Can you work these out from the model? Positions are in its coordinate system, mm. Face numbers are marked on the shaded views. A direction names the side the tool comes from. Coordinates: 2 decimals unless noted, no trailing zeros. Order: outer loops, then holes, each group sorted by start corner. A loop starts at its lowest first (then second) coordinate and runs counter-clockwise, first axis right, second up. Notation, with made-up numbers: (-2.5, 89) -> (20.5, 89) arc R34 ccw to (20.5, 125) -> close; hole circle Ø6 at (-34, 49). An arc over 180 degrees is marked (long way). Answer as CSV lines item,"result".
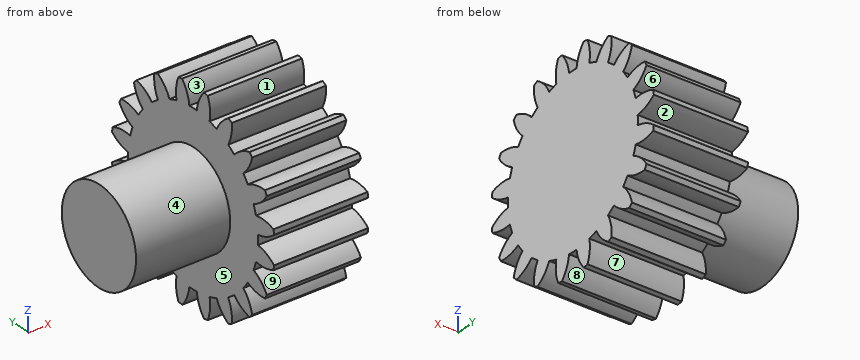
from build123d import *

# Parameters (mm, degrees)
BASPROSKE_W     = 10
BASPROSKE_H     = 11
TOOTHCUT_DEPTH  = 19.493242009
TEETHCUTS_COUNT = 20
TEETHCUTS_ANGLE = 342
BORSKE_R        = 0.5
BORE_DEPTH      = 50.0000508
SKETCH_1_R      = 5
EXTRUDE_1_DEPTH = 20


with BuildPart() as part:
    # BasProSke → Base-Revolve (revolve)
    with BuildSketch(Plane(origin=(0, 0, 0), x_dir=(1, 0, 0), z_dir=(0, 1, 0)), mode=Mode.PRIVATE) as base_revolve_sk:
        with Locations((5, 5.5)):
            Rectangle(BASPROSKE_W, BASPROSKE_H)
    revolve(base_revolve_sk.sketch.rotate(Axis((-10, 0, 0), (1, 0, 0)), 180), axis=Axis((-10, 0, 0), (1, 0, 0)))

    # TooCutSke → ToothCut (cut, through all)
    with BuildSketch(Plane(origin=(0, 0, 0), x_dir=(0, 0, -1), z_dir=(1, 0, 0))):
        with BuildLine():
            ThreePointArc((0.499924007, 8.734705318), (0, 8.749), (-0.499924007, 8.734705318))
            ThreePointArc((-0.499924007, 8.734705318), (-0.824302243, 9.905497836), (-1.485192705, 10.924909509))
            ThreePointArc((-1.485192705, 10.924909509), (0, 11.0254), (1.485192705, 10.924909509))
            ThreePointArc((1.485192705, 10.924909509), (0.824302243, 9.905497836), (0.499924007, 8.734705318))
        make_face()
    toothcut = extrude(amount=TOOTHCUT_DEPTH, mode=Mode.SUBTRACT)

    # TeethCuts: ToothCut ×20 about axis
    teethcuts_axis = Axis((-10, 0, 0), (1, 0, 0))
    for i in range(1, TEETHCUTS_COUNT):
        add(toothcut.rotate(teethcuts_axis, i * TEETHCUTS_ANGLE / (TEETHCUTS_COUNT - 1)), mode=Mode.SUBTRACT)

    # BorSke → Bore (cut, symmetric)
    with BuildSketch(Plane(origin=(0, 0, 0), x_dir=(0, 0, -1), z_dir=(1, 0, 0))):
        with Locations(Location((0, 0, 0), (0, 0, 180))):
            Circle(BORSKE_R)
    extrude(amount=BORE_DEPTH, both=True, mode=Mode.SUBTRACT)

    # 草图1 → 凸台-拉伸1 (add)
    with BuildSketch(Plane(origin=(10, 0, 0), x_dir=(0, 0, -1), z_dir=(1, 0, 0))):
        Circle(SKETCH_1_R)
    extrude(amount=-EXTRUDE_1_DEPTH)


solid = part.part
Q1. Which directions (+Z, -Z, +X, -X, +Y, -Y) give clear straight access to the entire face, cutting with the end or side of a thin tool? Please do the marked faces 5, 6, 7, 8 and 9.
Solution:
face 5,"-X"
face 6,"+X, -X, +Y"
face 7,"+X, -X"
face 8,"-Z, +X, -X"
face 9,"+X, -X, -Y"
Q2. Imagine slicing it at C-C (x = -3). List the corners of the cut face in (y, z) for me, and give its area (3 significant figures).
Solution:
outline,"circle Ø10 at (0, 0)"
area,"78.5 mm2"
Q3. For P1, Ø8, axis at x = 3.5, z = 5.5, coming from the -Y side; P2, Ø1.5, axis at y = -8.5, z = 3, coming from the -X side; P3, Ø2, axis at x = 0, z = -3.5, coming from the +Y side, each with a flat end and sliding along its axis, tell me the tip position at first contact or that it passes through.
Solution:
P1,"y = -10.9"
P2,"x = 0"
P3,"y = 9.75"
Q4. If I drill on line 1 (Z direction, x = 3.5, y = 9.5); line 2 (X direction, y = 3.5, z = 4.5), over which ranges is the centre line in solid material (lowest first)?
Solution:
line 1,"-5.24 to -4.19, -2.29 to -0.67, 0.67 to 2.29, 4.19 to 5.24"
line 2,"0 to 10"
Q5. We'd pull the mould along Y, two halves only. Please class the marked faces 1, 2, 3 and 4: pulls with the +Y half, pulls with the -Y half, needs draft (parallel to the pull), parting line crosses it, or undercut.
Solution:
face 1,"undercut"
face 2,"pulls with the +Y half"
face 3,"undercut"
face 4,"parting line crosses it"
Q6. Imagine slicing it at A-A (z = 0). List the corners of the cut face in (x, y) for me, and give its area (3 significant figures).
Solution:
outline,"(-10, -5) -> (0, -5) -> (0, -8.75) -> (10, -8.75) -> (10, 8.75) -> (0, 8.75) -> (0, 5) -> (-10, 5) -> close"
area,"275 mm2"
